Drawing for the job (mm, zero at the part's lowest x, y, z). A direction names the side the tool comes from. Round coordinates to 2 decimals unless told otherwise and drop trailing zeros. Loops run counter-clockwise (first coordinate to the right, second up) from the corner with the lowest first, then second, coordinate; pieces in that order, holes last. Notation, with made-up numbers: (-38.5, -40) - (-16.5, -40) arc R15 ccw to (-16.5, -30) - close; hole circle Ø2 at (56, 70.5). An arc over 180 degrees is marked (long way). Put each result on its own line as item: value.
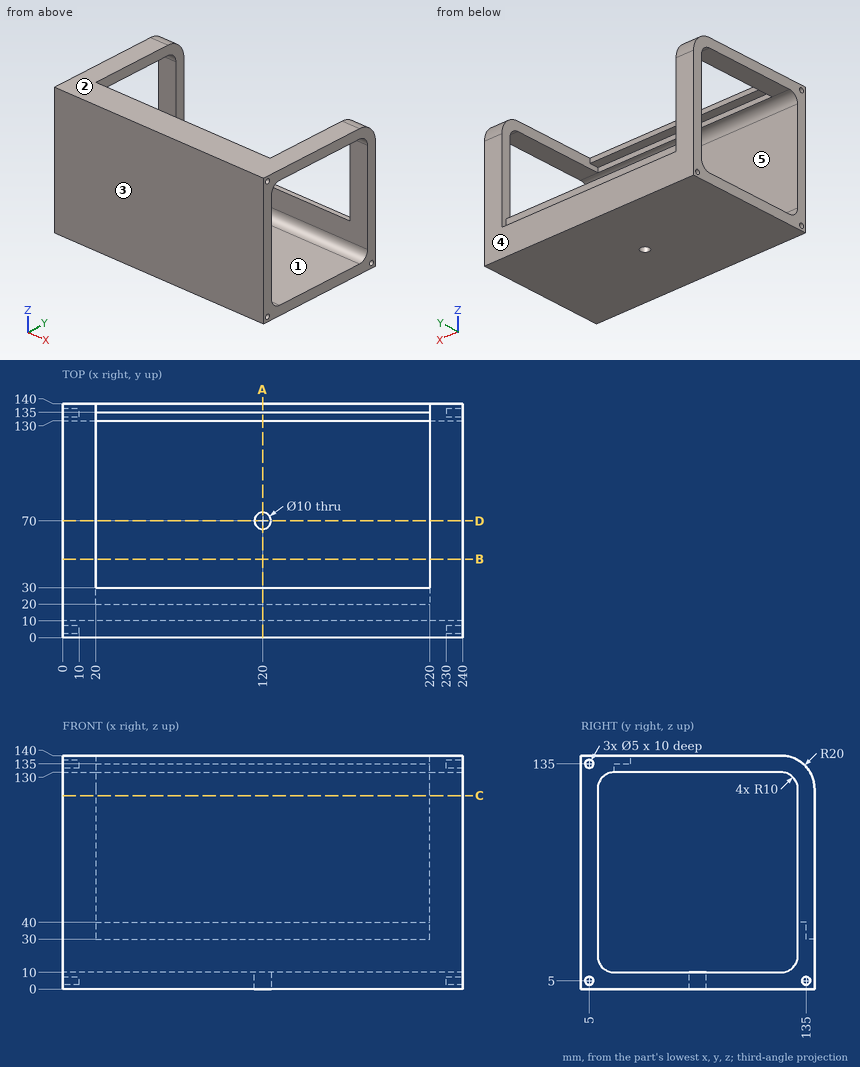
1. Band-saw the part on D-D (y = 70). List the corners of the cut face in (x, z).
A:
outline: (0, 0) - (115, 0) - (115, 10) - (0, 10) - close; (0, 130) - (20, 130) - (20, 140) - (0, 140) - close; (125, 0) - (240, 0) - (240, 10) - (125, 10) - close; (220, 130) - (240, 130) - (240, 140) - (220, 140) - close
2. Two-plate mould, pull along Y, no slides. Class the marked faces 1, 2 and 3: pulls with the +Y half, pulls with the -Y half, needs draft (parallel to the pull), parting line crosses it, or undercut.
A:
face 1: undercut
face 2: needs draft
face 3: pulls with the -Y half
3. Pin check, flat tips, straight feed: P1, Ø1.5, axis at y = 4.5, z = 134.5, coming from the +X side; P2, Ø10, axis at x = 82, y = 55.5, coming from the +Z side; P3, Ø1.5, axis at x = 164.5, z = 90.5, coming from the -Y side; P4, Ø10, axis at x = 202.5, z = 103.5, coming from the +Y side. Stop position of each tip, or through.
A:
P1: stops at x = 230
P2: stops at z = 10
P3: stops at y = 0
P4: stops at y = 10
4. Band-saw the part on B-B (y = 47). List the corners of the cut face in (x, z).
A:
outline: (0, 0) - (240, 0) - (240, 10) - (0, 10) - close; (0, 130) - (20, 130) - (20, 140) - (0, 140) - close; (220, 130) - (240, 130) - (240, 140) - (220, 140) - close
5. Tool access for the marked faces 4 and 5: list every direction of +Z, -Z, +X, -X, +Y, -Y with a clear straight run to the whole face (end or side of a thin tool).
A:
face 4: +Z, -Z, +X, -X, +Y
face 5: +X, -X
6. Probe line 1 along X through (y, z) = (130.5, 65.5); line 2 along Y through (x, z) = (187, 32); line 3 along Y through (x, z) = (31, 110.5). List the from-to ranges inside material, lowest first. Write a range as [from, to].
A:
line 1: x = [0, 20], [220, 240]
line 2: y = [0, 10], [130, 135]
line 3: y = [0, 10]
7. Band-saw the part on A-A (x = 120). List the corners of the cut face in (y, z).
A:
outline: (0, 0) - (65, 0) - (65, 10) - (20, 10) arc R10 cw to (10, 20) - (10, 120) arc R10 cw to (20, 130) - (20, 135) - (30, 135) - (30, 140) - (0, 140) - close; (75, 0) - (140, 0) - (140, 30) - (135, 30) - (135, 40) - (130, 40) - (130, 20) arc R10 cw to (120, 10) - (75, 10) - close
